```python
from build123d import *

# Parameters (mm, degrees)
SKETCH1_R           = 6.5
BOSS_EXTRUDE1_DEPTH = 6.5


with BuildPart() as part:
    # Sketch1 → Boss-Extrude1 (new body)
    with BuildSketch(Plane.XY):
        with Locations(Location((0, 0, 0), (0, 0, 180))):
            Circle(SKETCH1_R)
        with BuildLine():
            Line((5.2, -1.5), (3.708099244, -1.5))
            ThreePointArc((3.708099244, -1.5), (-4, 0), (3.708099244, 1.5))
            Line((3.708099244, 1.5), (5.2, 1.5))
            Line((5.2, 1.5), (5.2, -1.5))
        make_face(mode=Mode.SUBTRACT)
    extrude(amount=BOSS_EXTRUDE1_DEPTH)


solid = part.part
```
Input: part model. Units: mm. Frame: model coordinates. A direction names the side the tool comes from. Coordinates: 2 decimals unless noted, no trailing zeros. Loops run counter-clockwise (first coordinate to the right, second up) from the corner with the lowest first, then second, coordinate; pieces in that order, holes last. Notation, with made-up numbers: M 35,61.5 L 66,61.5 A25 ccw 66,75.5 Z; hole C 80,70 d3. An arc over 180 degrees is marked long. One line per item, written item: value.
(1) Pin query (flat end, axial travel): pin 1 (1.5 mm diameter, centred on y = 3.5, z = 5.5, fed in from +X); pin 2 (1.2 mm diameter, centred on x = 4.5, z = 3.5, fed in from -Y); pin 3 (1 mm diameter, centred on y = -1, z = 5.5, fed in from +X). Return the tip coordinate at first contact, or that it passes through.
Filled in:
pin 1: x = 5.89
pin 2: y = -5.2
pin 3: x = 6.48
(2) Line query: line 1 along Y through (x, z) = (0, 0.5); line 2 along X through (y, z) = (-0.25, 3.25); line 3 along X through (y, z) = (-1.75, 4.25). Output: solid intervals per line, ascending. Write a range as from..to.
Filled in:
line 1: -6.5..-4, 4..6.5
line 2: -6.5..-3.99, 5.2..6.5
line 3: -6.26..-3.6, 3.6..6.26
(3) Reachability of faces 1 (the flat face through (5.2, 0, 3)), 2 (the flat face through (-4.2, -0.1, 6.5)) from +Z, -Z, +X, -X, +Y, -Y: full face, straight path, thin tool, end or side. Return the list, or none.
Filled in:
face 1: +Z, -Z
face 2: +Z, +X, -X, +Y, -Y
(4) Section A-A (y = 0). Output: boundary loops of the cut face in (x, z), and give its area (3 significant figures).
Filled in:
outline: M -6.5,0 L -4,0 L -4,6.5 L -6.5,6.5 Z; M 5.2,0 L 6.5,0 L 6.5,6.5 L 5.2,6.5 Z
area: 24.7 mm^2
(5) Section B-B (x = 0). Output: boundary loops of the cut face in (y, z).
Filled in:
outline: M -6.5,0 L -4,0 L -4,6.5 L -6.5,6.5 Z; M 4,0 L 6.5,0 L 6.5,6.5 L 4,6.5 Z
(6) Pull-direction query (Y, two-part tool) for faces 3 (the cylindrical face through (-4, 0, 3)), 4 (the flat face through (-4.2, -0.1, 0)), 5 (the cylindrical face through (5.158, 3.955, 3.204)); classes: +Y half, -Y half, draft (parallel to the pull), parting line (faces both ways), or undercut.
Filled in:
face 3: undercut
face 4: draft
face 5: parting line
(7) Section D-D (x = -5.5). Output: boundary loops of the cut face in (y, z), and give its area (3 significant figures).
Filled in:
outline: M -3.46,0 L 3.46,0 L 3.46,6.5 L -3.46,6.5 Z
area: 45.0 mm^2
(8) Section C-C (z = 6). Output: boundary loops of the cut face in (x, y), and give its area (3 significant figures).
Filled in:
outline: C 0,0 d13; hole M 3.71,-1.5 L 5.2,-1.5 L 5.2,1.5 L 3.71,1.5 A4 ccw long Z
area: 78.6 mm^2
